Input: part model. Units: mm. Frame: model coordinates. Face numbers are marked on the shaded views. A direction names the side the tool comes from. Coordinates: 2 decimals unless noted, no trailing zeros. Loops run counter-clockwise (first coordinate to the right, second up) from the corner with the lowest first, then second, coordinate; pieces in that order, holes last.
Item 1: Section A-A on y = 27.5. Return loops of the section in (x, z).
Item 2: Pull-direction query (X, two-part tool) for the marked faces 3, 4 and 5; classes: released by +X, released by -X, zero draft, split by the parting line, or undercut.
Item 3: Section B-B on x = -22. Return loops of the section in (y, z).
Item 4: Contact query for flat-ended pins moving along their axis: P1, Ø6, axis at x = -1.5, z = 16.5, coming from the -Y side; P2, Ø7, axis at x = -5.5, z = -4, coming from the +Y side; P3, Ø3, axis at x = -23, z = -2, coming from the +Y side. Output: stop coordinate, or through.
Item 5: Section D-D on x = 0. Return loops of the section in (y, z), and give its area (3 significant figures).
Item 6: Ray query, line 1 along X through (y, z) = (26.25, 0); line 2 along Y through (x, z) = (-25, 13.5); line 3 along Z through (x, y) = (-9, 23.5). Return the intervals inside material, ascending.
Item 7: Reachability of the marked faces 1 and 2 from +Z, -Z, +X, -X, +Y, -Y: full face, straight path, thin tool, end or side. Return the list, or none.
Item 8: Section C-C on z = 14. Return loops of the section in (x, y), and give its area (3 significant figures).
```python
from build123d import *

# Parameters (mm, degrees)
ESQUISSE1_W             = 42
ESQUISSE1_H             = 42
BOSS_EXTRU_1_DEPTH      = 30
ESQUISSE2_R             = 12
ENL_V_MAT_EXTRU_1_DEPTH = 8
ESQUISSE4_W             = 42
ESQUISSE4_H             = 30
BOSS_EXTRU_3_DEPTH      = 16
ESQUISSE5_W             = 6
ESQUISSE5_H             = 13
ENL_V_MAT_EXTRU_2_DEPTH = 11
ESQUISSE6_W             = 5.949379811
ESQUISSE6_H             = 6
ENL_V_MAT_EXTRU_3_DEPTH = 56.00227268


with BuildPart() as part:
    # Esquisse1 → Boss.-Extru.1 (new body)
    with BuildSketch(Plane(origin=(0, 0, 0), x_dir=(1, 0, 0), z_dir=(0, 1, 0))):
        Rectangle(ESQUISSE1_W, ESQUISSE1_H)
    extrude(amount=BOSS_EXTRU_1_DEPTH)

    # Esquisse2 → Enlèv. mat.-Extru.1 (cut)
    with BuildSketch(Plane(origin=(0, 30, 0), x_dir=(1, 0, 0), z_dir=(0, 1, 0))):
        with Locations(Location((0, 0, 0), (0, 0, 270))):
            Circle(ESQUISSE2_R)
    extrude(amount=-ENL_V_MAT_EXTRU_1_DEPTH, mode=Mode.SUBTRACT)

    # Esquisse4 → Boss.-Extru.3 (add)
    with BuildSketch(Plane.ZY.offset(21)):
        with Locations((0, 15)):
            Rectangle(ESQUISSE4_W, ESQUISSE4_H)
    extrude(amount=BOSS_EXTRU_3_DEPTH)

    # Esquisse5 → Enlèv. mat.-Extru.2 (cut)
    with BuildSketch(Plane(origin=(0, 30, 0), x_dir=(1, 0, 0), z_dir=(0, 1, 0))):
        with Locations((-24, 0)):
            Rectangle(ESQUISSE5_W, ESQUISSE5_H)
    extrude(amount=-ENL_V_MAT_EXTRU_2_DEPTH, mode=Mode.SUBTRACT)

    # Esquisse6 → Enlèv. mat.-Extru.3 (cut, through all)
    with BuildSketch(Plane.XY.offset(-6.5)):
        with Locations((-23.974689906, 23.009155876)):
            Rectangle(ESQUISSE6_W, ESQUISSE6_H)
    extrude(amount=ENL_V_MAT_EXTRU_3_DEPTH, mode=Mode.SUBTRACT)


solid = part.part
```
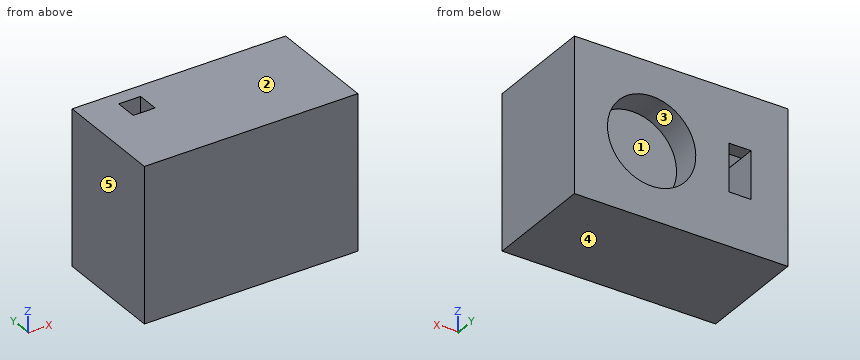
Results found:
1. outline: (-37, -21) - (21, -21) - (21, 21) - (-37, 21) - close; hole (-27, -6.5) - (-21, -6.5) - (-21, 6.5) - (-27, 6.5) - close; hole circle Ø24 at (0, 0)
2. face 3: undercut
2. face 4: zero draft
2. face 5: released by -X
3. outline: (0, -21) - (30, -21) - (30, -6.5) - (19, -6.5) - (19, 6.5) - (20.01, 6.5) - (20.01, 21) - (0, 21) - close; (26.01, 6.5) - (30, 6.5) - (30, 21) - (26.01, 21) - close
4. P1: stops at y = 0
4. P2: stops at y = 22
4. P3: stops at y = 19
5. outline: (0, -21) - (30, -21) - (30, -12) - (22, -12) - (22, 12) - (30, 12) - (30, 21) - (0, 21) - close
5. area: 1,070 mm2
6. line 1: x = -37 to -27, -21 to -12, 12 to 21
6. line 2: y = 0 to 20.01, 26.01 to 30
6. line 3: z = -21 to -7.94, 7.94 to 21
7. face 1: +Y
7. face 2: +Z, +X, -X, +Y, -Y
8. outline: (-37, 0) - (21, 0) - (21, 30) - (-37, 30) - close; hole (-26.95, 20.01) - (-21, 20.01) - (-21, 26.01) - (-26.95, 26.01) - close
8. area: 1,700 mm2
